```python
from build123d import *

# Parameters (mm, degrees)
CUT_EXTRUDE1_DEPTH      = 12.554003635
CUT_EXTRUDE1_DEPTH_BACK = 12.554003635
SKETCH2_W               = 1.25
SKETCH2_H               = 1.2
CHAMFER1_SIZE           = 0.42
CHAMFER1_SIZE2          = 0.727461339


with BuildPart() as part:
    # Sketch1 → Revolve1 (revolve)
    with BuildSketch(Plane.XY, mode=Mode.PRIVATE) as revolve1_sk:
        Polygon((0, 4.65), (0.25, 4.65), (2.8, 2.1), (9.5, 2.1), (9.5, 0), (0, 0), align=None)
    revolve(revolve1_sk.sketch.rotate(Axis((6.620684694, 0, 0), (-1, 0, 0)), 90), axis=Axis((6.620684694, 0, 0), (-1, 0, 0)))

    # Sketch2 → Cut-Extrude1 (cut, two sides: drawn at the far end of the back side and taken through both)
    with BuildSketch(Plane.XY.offset(-CUT_EXTRUDE1_DEPTH_BACK)):
        with Locations((0.625, 0)):
            Rectangle(SKETCH2_W, SKETCH2_H)
    extrude(amount=CUT_EXTRUDE1_DEPTH + CUT_EXTRUDE1_DEPTH_BACK, mode=Mode.SUBTRACT)

    # Chamfer1
    chamfer1_edges = [part.edges().sort_by_distance(p)[0] for p in [
        (9.5, 0, 2.1),
    ]]
    chamfer1_side = [part.faces().sort_by_distance(p)[0] for p in [
        (9.5, 0, 0),
    ]]
    chamfer(chamfer1_edges, length=CHAMFER1_SIZE, length2=CHAMFER1_SIZE2, reference=chamfer1_side[0])


solid = part.part
```
CAD build for the part. Positions are in the model's coordinates, mm. A direction names the side the tool comes from. Round coordinates to 2 decimals unless told otherwise and drop trailing zeros. Write each loop counter-clockwise with the first axis right and the second up, starting at its lowest first coordinate (ties: lowest second). Pieces come first, ordered by that corner, then holes. Notation, with made-up numbers: M -23,-34.75 L 35,-34.75 A25 cw 35,-2.75 Z; hole C 66.25,70.25 d5. An arc over 180 degrees is marked long. One line per question, with ' | ' between items.
1. Mould opens along Y. For faces 1 (the flat face through (1, -0.6, 0)), 2 (the cylindrical face through (5.828, -0.631, -2.003)), 3 (the flat face through (1.25, 0, 0)), 4 (the flat face through (9.5, 0, 0)) say: pulls with the +Y half, pulls with the -Y half, needs draft (parallel to the pull), parting line crosses it, or undercut.
Working result:
face 1: undercut | face 2: parting line crosses it | face 3: undercut | face 4: needs draft
2. Cut at D-D on x = 2.25. Write the cut outline in (y, z), and give its area (3 significant figures).
Working result:
outline: C 0,0 d5.3 | area: 22.1 mm2
3. Probe L1, parallel to Y at x = 5.75, z = 0; L2, parallel to Y at x = 0.5, z = 4; L3, parallel to X at y = 3.75, z = -1.25. List the from-to ranges inside material, lowest first. Write a range as from..to.
Working result:
L1: -2.1..2.1 | L2: -1.83..-0.6, 0.6..1.83 | L3: 0..0.95
4. Cut at A-A on z = 0. Write the cut outline in (x, y).
Working result:
outline: M 0,-4.65 L 0.25,-4.65 L 2.8,-2.1 L 8.77,-2.1 L 9.5,-1.68 L 9.5,1.68 L 8.77,2.1 L 2.8,2.1 L 0.25,4.65 L 0,4.65 L 0,0.6 L 1.25,0.6 L 1.25,-0.6 L 0,-0.6 Z
5. Pin check, flat tips, straight feed: pin 1 Ø4 at (x, z) = (5.5, -3) entering from +Y; pin 2 Ø1 at (y, z) = (0, -1.5) entering from -X; pin 3 Ø3 at (x, y) = (7, 0.5) entering from +Z. Stop position of each tip, or through.
Working result:
pin 1: y = 1.85 | pin 2: x = 1.25 | pin 3: z = 2.1
6. Which spindle directions (+Z, -Z, +X, -X, +Y, -Y) get a long thin tool onto all of the face, cutting with end or side? Do faces 5 (the flat face through (1, 0.6, 0)), 6 (the flat face through (0, -2, 0)). Say none if no direction does.
Working result:
face 5: +Z, -Z, -X | face 6: +Z, -Z, -X, +Y, -Y
7. Cut at C-C on x = 3.5. Write the cut outline in (y, z), and give its area (3 significant figures).
Working result:
outline: C 0,0 d4.2 | area: 13.9 mm2
8. Cut at B-B on y = 0. Write the cut outline in (x, z), and give its area (3 significant figures).
Working result:
outline: M 1.25,-3.65 L 2.8,-2.1 L 8.77,-2.1 L 9.5,-1.68 L 9.5,1.68 L 8.77,2.1 L 2.8,2.1 L 1.25,3.65 Z | area: 36.7 mm2
